Check sheet for the modelled part. Datum: model origin and axes. Units: mm. Round coordinates to 2 decimals unless told otherwise and drop trailing zeros. Order: outer loops, then holes, each group sorted by start corner. A loop starts at its lowest first (then second) coordinate and runs counter-clockwise, first axis right, second up. Notation, with made-up numbers: M 35,73.25 L 84,73.25 A14 ccw 84,98.25 Z; hole C -8,46 d7. An arc over 180 degrees is marked long. One line per item, written item: value. Start each with the question number.
(1) Cross-section at C-C, the plane z = 1.5. Enter the section's corners in (x, y), and give its area (3 significant figures).
(2) Cross-section at D-D, the plane z = -1.75. Count the separate pieces of the cut face and the enclosed holes in it, and give its area (3 significant figures).
(3) Cross-section at A-A, the plane z = 0.75. Enter the section's corners in (x, y), and give its area (3 significant figures).
(4) Thickness scan on L1, parallel to Y at x = 0.05, z = -2; L2, parallel to Y at x = 0.1, z = -1.25; L3, parallel to Y at x = 0, z = 2.25. Record the ranges inside material, lowest first.
(5) Cross-section at B-B, the plane y = -1.25. Enter the section's corners in (x, z), and give its area (3 significant figures).
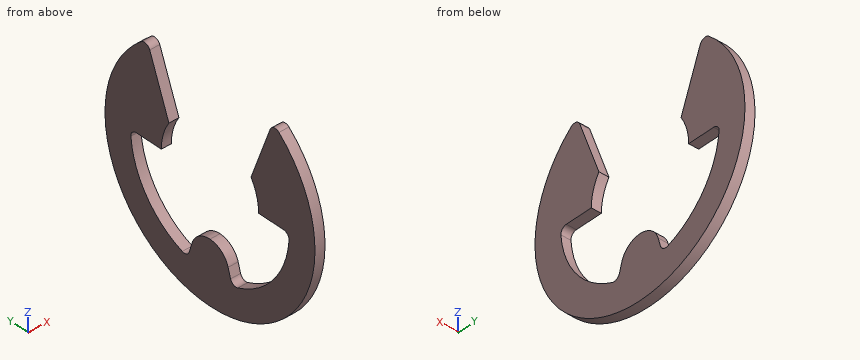
from build123d import *

# Parameters (mm, degrees)
EXTRUDE1_DEPTH = 0.15
FILLET1_R      = 0.18
FILLET2_START  = -1
FILLET2_DEPTH  = 2


with BuildPart() as part:
    # Sketch1 → Extrude1 (new, symmetric)
    with BuildSketch(Plane(origin=(0, 0, 0), x_dir=(0, 0, -1), z_dir=(1, 0, 0))):
        with BuildLine():
            Line((-2.761953542, -2.067392713), (-0.858778202, -1.35))
            ThreePointArc((-0.858778202, -1.35), (-0.447213595, -1.53622915), (0, -1.6))
            Line((0, -1.6), (0, -2.606451613))
            ThreePointArc((0, -2.606451613), (1.564404659, -2.084760915), (2.50256684, -0.728525373))
            Line((2.50256684, -0.728525373), (1.53622915, -0.447213595))
            ThreePointArc((1.53622915, -0.447213595), (1.6, 0), (1.53622915, 0.447213595))
            Line((1.53622915, 0.447213595), (2.50256684, 0.728525373))
            ThreePointArc((2.50256684, 0.728525373), (1.564404659, 2.084760915), (0, 2.606451613))
            Line((0, 2.606451613), (0, 1.6))
            ThreePointArc((0, 1.6), (-0.447213595, 1.53622915), (-0.858778202, 1.35))
            Line((-0.858778202, 1.35), (-2.761953542, 2.067392713))
            ThreePointArc((-2.761953542, 2.067392713), (3.45, 0), (-2.761953542, -2.067392713))
        make_face()
    extrude(amount=EXTRUDE1_DEPTH, both=True)

    # Fillet1
    fillet1_edges = [part.edges().sort_by_distance(p)[0] for p in [
        (0, -2.067392713, 2.761953542),
        (0, -2.606451613, 0),
        (0, -0.728525373, -2.50256684),
        (0, 0.728525373, -2.50256684),
        (0, 2.606451613, 0),
        (0, 2.067392713, 2.761953542),
    ]]
    fillet(fillet1_edges, radius=FILLET1_R)

    # Fillet2: read off the stored shape, not the designer's step
    # Fillet2 outline → Fillet2 (cut)
    with BuildSketch(Plane.YZ.offset(FILLET2_START)):
        with BuildLine():
            Line((-0.447213595, -1.53622915), (-0.595966919, -2.047213595))
            add(Edge.make_bspline(
                [(-0.595966919, -2.047213595), (-0.522890719, -1.796188606), (-0.310518672, -1.6), (0, -1.6)],
                knots=[0, 0, 0, 0, 0.5, 0.5, 0.5, 0.5], degree=3, weights=[1, 0.759836166, 0.639754249, 0.639754249]))
            ThreePointArc((0, -1.6), (-0.225868723, -1.583977058), (-0.447213595, -1.53622915))
        make_face()
        with BuildLine():
            ThreePointArc((0.447213595, -1.53622915), (0.225868723, -1.583977058), (0, -1.6))
            add(Edge.make_bspline(
                [(0, -1.6), (0.310518672, -1.6), (0.522890719, -1.796188606), (0.595966919, -2.047213595)],
                knots=[0.5, 0.5, 0.5, 0.5, 1, 1, 1, 1], degree=3, weights=[0.639754249, 0.639754249, 0.759836166, 1]))
            Line((0.595966919, -2.047213595), (0.447213595, -1.53622915))
        make_face()
    extrude(amount=FILLET2_DEPTH, mode=Mode.SUBTRACT)


solid = part.part
Values found:
1. outline: M -0.15,-3.11 L 0.15,-3.11 L 0.15,-1.59 L -0.15,-1.59 Z; M -0.15,1.59 L 0.15,1.59 L 0.15,3.11 L -0.15,3.11 Z
1. area: 0.909 mm^2
2. separate pieces: 3
2. enclosed holes: 0
2. area: 0.868 mm^2
3. outline: M -0.15,-3.37 L 0.15,-3.37 L 0.15,-1.41 L -0.15,-1.41 Z; M -0.15,1.41 L 0.15,1.41 L 0.15,3.37 L -0.15,3.37 Z
3. area: 1.17 mm^2
4. L1: -2.81 to -1.67, -0.58 to 0.58, 1.67 to 2.81
4. L2: -3.22 to -2.29, 2.29 to 3.22
4. L3: -2.62 to -1.87, 1.87 to 2.62
5. outline: M -0.15,-3.22 L 0.15,-3.22 L 0.15,-2.29 L -0.15,-2.29 Z
5. area: 0.279 mm^2
